from build123d import *

# Parameters (mm, degrees)
SKETCH2_W           = 177.8
SKETCH2_H           = 101.6
SKETCH2_W_2         = 152.4
SKETCH2_H_2         = 76.2
BOSS_EXTRUDE2_DEPTH = 2600
SKETCH1_R           = 38.1
BOSS_EXTRUDE3_DEPTH = 44.45
BOSS_EXTRUDE5_START = -44.45
SKETCH3_R           = 38.1
BOSS_EXTRUDE5_DEPTH = 44.45
FILLET1_R           = 12.7
FILLET2_R           = 12.7
SKETCH5_R           = 12.7
BOSS_EXTRUDE7_DEPTH = 19.05
LPATTERN1_COUNT     = 2
LPATTERN1_PITCH     = 165.1


with BuildPart() as part:
    # Sketch2 → Boss-Extrude2 (new body)
    with BuildSketch(Plane.XY):
        with Locations((-88.9, 50.8)):
            Rectangle(SKETCH2_W, SKETCH2_H)
        with Locations((-88.9, 50.8)):
            Rectangle(SKETCH2_W_2, SKETCH2_H_2, mode=Mode.SUBTRACT)
    extrude(amount=BOSS_EXTRUDE2_DEPTH)

    # Sketch1 → Boss-Extrude3 (add)
    with BuildSketch(Plane(origin=(0, 0, 0), x_dir=(0, 0, -1), z_dir=(1, 0, 0))):
        with BuildLine():
            Line((-127, 101.6), (0, 101.6))
            Line((0, 101.6), (0, 304.8))
            ThreePointArc((0, 304.8), (-55.382017361, 361.922646449), (-114.190611982, 308.334272869))
            Line((-114.190611982, 308.334272869), (-127, 101.6))
        make_face()
        with Locations((-57.15, 304.8)):
            Circle(SKETCH1_R, mode=Mode.SUBTRACT)
    extrude(amount=-BOSS_EXTRUDE3_DEPTH)

    # Sketch3 → Boss-Extrude5 (add)
    with BuildSketch(Plane.ZY.offset(177.8).offset(BOSS_EXTRUDE5_START)):
        with BuildLine():
            Line((0, 304.8), (0, 101.6))
            Line((0, 101.6), (127, 101.6))
            Line((127, 101.6), (114.190611982, 308.334272869))
            ThreePointArc((114.190611982, 308.334272869), (55.382017361, 361.922646449), (0, 304.8))
        make_face()
        with Locations(Location((57.15, 304.8, 0), (0, 0, 180))):
            Circle(SKETCH3_R, mode=Mode.SUBTRACT)
    extrude(amount=BOSS_EXTRUDE5_DEPTH)

    # Fillet1
    fillet1_edges = [part.edges().sort_by_distance(p)[0] for p in [
        (-12.7, 88.9, 1300),
        (-165.1, 88.9, 1300),
        (-165.1, 12.7, 1300),
        (-12.7, 12.7, 1300),
    ]]
    fillet(fillet1_edges, radius=FILLET1_R)

    # Fillet2
    fillet2_edges = [part.edges().sort_by_distance(p)[0] for p in [
        (-44.45, 101.6, 63.5),
        (-22.225, 101.6, 127),
        (-133.35, 101.6, 63.5),
        (-155.575, 101.6, 127),
    ]]
    fillet(fillet2_edges, radius=FILLET2_R)

    # Sketch5 → Boss-Extrude7 (add)
    with BuildSketch(Plane(origin=(0, 0, 0), x_dir=(0, 0, -1), z_dir=(1, 0, 0))):
        with BuildLine():
            Line((-2600, 101.6), (-2600, 180.34))
            ThreePointArc((-2600, 180.34), (-2583.812295525, 199.173740052), (-2562.760129729, 185.999604185))
            Line((-2562.760129729, 185.999604185), (-2536.5, 101.6))
            Line((-2536.5, 101.6), (-2600, 101.6))
        make_face()
        with Locations((-2580.95, 180.34)):
            Circle(SKETCH5_R, mode=Mode.SUBTRACT)
    boss_extrude7 = extrude(amount=-BOSS_EXTRUDE7_DEPTH)

    # LPattern1: Boss-Extrude7 ×2
    with Locations(*[(-i * LPATTERN1_PITCH, 0, 0) for i in range(1, LPATTERN1_COUNT)]):
        add(boss_extrude7)


solid = part.part
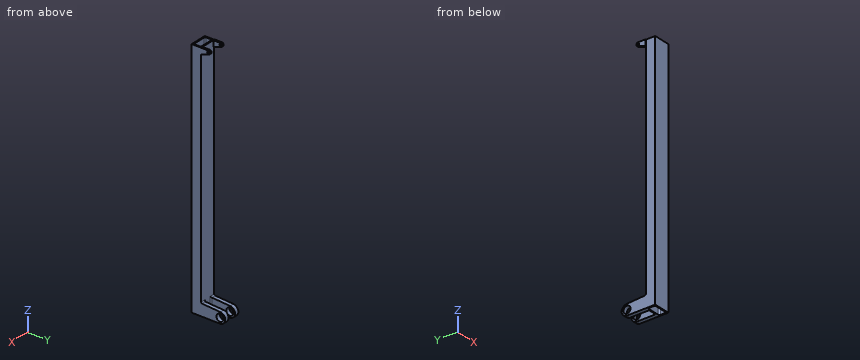
Could you check a few things on this model? Use its own coordinates, in mm. Give positions to 0.01 mm unless a question says otherwise; leave off trailing zeros. Order: outer loops, then holes, each group sorted by start corner. A loop starts at its lowest first (then second) coordinate and runs counter-clockwise, first axis right, second up.
Item 1: I need wall thicknesses on line 1 (Y direction, x = -30.5, z = 57.15); line 2 (X direction, y = 79, z = 1140.5); line 3 (Y direction, x = -173.25, z = 2580.95). Which ranges of each line are inside material? Lowest first, please.
Item 2: If we section it at A-A, the plane z = 57.15: Write out the boundary of the cut face in (x, y).
Item 3: If we section it at B-B, the plane x = -86: Write out the boundary of the cut face in (y, z), plus the area to 3 significant figures.
Item 4: If we section it at C-C, the plane z = 1029: Write out the boundary of the cut face in (x, y).
Item 5: I'm going to push flat-ended pins straight in: pin 1 (15 mm diameter, centred on y = 63.5, z = 987.5, fed in from -X); pin 2 (1.9 mm diameter, centred on x = -179.5, z = 2575.5, fed in from -Y). Where does each tip first touch, or does it pass through?
Values:
1. line 1: y = 0 to 12.7, 88.9 to 266.7, 342.9 to 361.95
1. line 2: x = -177.8 to -164.79, -13.01 to 0
1. line 3: y = 0 to 167.64, 193.04 to 199.39
2. outline: (-177.8, 0) - (0, 0) - (0, 266.7) - (-44.45, 266.7) - (-44.45, 114.3) arc R12.7 cw to (-57.15, 101.6) - (-120.65, 101.6) arc R12.7 cw to (-133.35, 114.3) - (-133.35, 266.7) - (-177.8, 266.7) - close; (-177.8, 342.9) - (-133.35, 342.9) - (-133.35, 361.95) - (-177.8, 361.95) - close; (-44.45, 342.9) - (0, 342.9) - (0, 361.95) - (-44.45, 361.95) - close; hole (-165.1, 25.4) arc R12.7 ccw to (-152.4, 12.7) - (-25.4, 12.7) arc R12.7 ccw to (-12.7, 25.4) - (-12.7, 76.2) arc R12.7 ccw to (-25.4, 88.9) - (-152.4, 88.9) arc R12.7 ccw to (-165.1, 76.2) - close
3. outline: (0, 0) - (12.7, 0) - (12.7, 2600) - (0, 2600) - close; (88.9, 0) - (101.6, 0) - (101.6, 2600) - (88.9, 2600) - close
3. area: 66,000 mm2
4. outline: (-177.8, 0) - (0, 0) - (0, 101.6) - (-177.8, 101.6) - close; hole (-165.1, 25.4) arc R12.7 ccw to (-152.4, 12.7) - (-25.4, 12.7) arc R12.7 ccw to (-12.7, 25.4) - (-12.7, 76.2) arc R12.7 ccw to (-25.4, 88.9) - (-152.4, 88.9) arc R12.7 ccw to (-165.1, 76.2) - close
5. pin 1: stops at x = -177.8
5. pin 2: stops at y = 101.6
